The model under review builds one solid part; all positions refer to its coordinate system, in mm. A direction names the side the tool comes from. Round coordinates to 2 decimals unless told otherwise and drop trailing zeros. Order: outer loops, then holes, each group sorted by start corner. A loop starts at its lowest first (then second) coordinate and runs counter-clockwise, first axis right, second up. Notation, with made-up numbers: M 72,-8.75 L 80,-8.75 A26 cw 80,11.25 Z; hole C 39.5,6.5 d11. An arc over 180 degrees is marked long. Answer as a JSON object with one key per item and string values. Group by question number.
1. Add section B-B on y = 4. State the section outline as (x, z) points.
2. To check wall thickness, follow probe 1 along Y at (x, z) = (-0.5, -3); probe 2 along Y at (x, z) = (-3, 2); probe 3 along X at (y, z) = (5.25, 0). State the ranges of each line that lie inside material, in increasing order. Write a range as [from, to].
3. Machinability: for faces 5 (the face through (2.056, 1.09, 2.681)), 6 (the face through (3.47, 10.38, 0.77)), which of the approach directions +Z, -Z, +X, -X, +Y, -Y give a long, thin tool a straight path to every point of the face, cutting with its end or side? Answer none if there is none.
4. Mouldability with a two-part tool opening along Z and no side actions: class faces 1 (the face through (-2.556, 15.143, 0.336)), 2 (the face through (-1.95, 0.36, 3.45)), 3 (the face through (-1.924, 5.474, 0.253)), 4 (the face through (3, 0.711, -2)) as released by +Z, released by -Z, zero draft, split by the parting line, or undercut.
5. Clearance check with flat-ended pins moving along their axes: P1, Ø1, axis at x = 0, y = 13, coming from the +Z side; P2, Ø3.5, axis at x = -0.5, z = 1, coming from the -Y side; P3, Ø4, axis at y = 7, z = 0.5, coming from the +X side; P4, Ø2, axis at x = 0.5, z = -0.5, coming from the -Y side. State where each tip first meets the part, or that it passes through.
6. Add section D-D on y = 13. State the section outline as (x, z) points.
```python
from build123d import *

# Parameters (mm, degrees)
HEXDIESKE_R  = 4.609084
HEXDIE_DEPTH = 0.7112


with BuildPart() as part:
    # BodySke → Body (revolve)
    with BuildSketch(Plane.XY, mode=Mode.PRIVATE) as body_sk:
        Polygon((3.556, 0), (4.596384, 0), (4.596384, 0.7112), (3.3782, 0.7112), (3.3782, 1.45796), (3.556, 1.45796), (3.556, 19.05), (1.94056, 19.05), (1.94056, 0.00508), (0, 0.00508), (0, 0.00254), (3.556, 0.00254), align=None)
    revolve(body_sk.sketch.rotate(Axis((0, 0, 0), (0, 1, 0)), 90), axis=Axis((0, 0, 0), (0, 1, 0)))

    # TapDriSke → TapDrill (revolve, cut)
    with BuildSketch(Plane.XY, mode=Mode.PRIVATE) as tapdrill_sk:
        Polygon((1.94056, -3.95732), (1.94056, 19.05), (0, 19.05), (0, -4.761126271), align=None)
    revolve(tapdrill_sk.sketch.rotate(Axis((0, 0, 0), (0, 1, 0)), 90), axis=Axis((0, 0, 0), (0, 1, 0)), mode=Mode.SUBTRACT)

    # EndChamferSke → EndChamfer (revolve, cut)
    with BuildSketch(Plane.XY, mode=Mode.PRIVATE) as endchamfer_sk:
        Polygon((2.5781, 11.1252), (2.5781, 19.304), (1.94056, 19.304), (1.94056, 10.79451682), (2.413, 11.1252), align=None)
    revolve(endchamfer_sk.sketch.rotate(Axis((0, -2.54, 0), (0, 1, 0)), 90), axis=Axis((0, -2.54, 0), (0, 1, 0)), mode=Mode.SUBTRACT)

    # HexDieSke → HexDie (cut)
    with BuildSketch(Plane(origin=(0, 0.7112, 0), x_dir=(-1, 0, 0), z_dir=(0, 1, 0))):
        Circle(HEXDIESKE_R)
        Polygon((0, 4.575385413), (3.9624, 2.287692707), (3.9624, -2.287692707), (0, -4.575385413), (-3.9624, -2.287692707), (-3.9624, 2.287692707), align=None, mode=Mode.SUBTRACT)
    extrude(amount=-HEXDIE_DEPTH, mode=Mode.SUBTRACT)


solid = part.part
```
Recorded:
{
 "1": {"outline": "C 0,0 d7.11; hole C 0,0 d3.88"},
 "2": {"probe 1": "y = [0, 19.05]", "probe 2": "y = [0, 0.71]", "probe 3": "x = [-3.56, -1.94], [1.94, 3.56]"},
 "3": {"face 5": "none", "face 6": "+Y"},
 "4": {"face 1": "undercut", "face 2": "released by +Z", "face 3": "undercut", "face 4": "zero draft"},
 "5": {"P1": "stops at z = 3.56", "P2": "stops at y = 0", "P3": "stops at x = 3.56", "P4": "passes through"},
 "6": {"outline": "C 0,0 d7.11; hole C 0,0 d5.16"}
}
